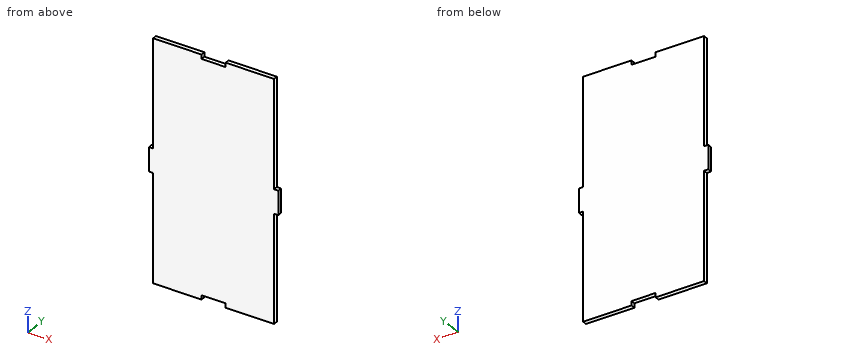
from build123d import *

# Parameters (mm, degrees)
F0_W     = 2.7432
F0_H     = 15.24
F1_DEPTH = 2.7432


with BuildPart() as f1:
    # F0 (on Front) → F1 (new body)
    with BuildSketch(Plane.XZ):
        Polygon((-7.62, 84.245604), (-38.1, 84.245604), (-38.1, 15.665604), (-38.1, 0.425604), (-38.1, -68.154396), (-7.62, -68.154396), (-7.62, -65.411196), (7.62, -65.411196), (7.62, -68.154396), (38.1, -68.154396), (38.1, 0.425604), (38.1, 15.665604), (38.1, 84.245604), (7.62, 84.245604), (7.62, 81.502404), (-7.62, 81.502404), align=None)
        with Locations((-39.4716, 8.045604)):
            Rectangle(F0_W, F0_H)
        with Locations((39.4716, 8.045604)):
            Rectangle(F0_W, F0_H)
    extrude(amount=F1_DEPTH)


solid = f1.part
Model file for the job. Use its own axes, mm. Give positions to 0.01 mm unless a question says otherwise; leave off trailing zeros. Write each loop counter-clockwise with the first axis right and the second up, starting at its lowest first coordinate (ties: lowest second). Pieces come first, ordered by that corner, then holes. Notation, with made-up numbers: M 62.25,0 L 71.25,0 A19 ccw 71.25,26 Z; hole C 38,13.5 d2. An arc over 180 degrees is marked long. One line per item, written item: value. Start each with the question number.
Q1. Drop flat-ended pins along their axis: pin 1 Ø1.5 at (y, z) = (-0.5, 65.5) entering from +X; pin 2 Ø1 at (y, z) = (-1.5, -25) entering from -X; pin 3 Ø1.4 at (x, y) = (39, -2) entering from +Z. Give the stop position or say it passes through.
Q2. Probe probe 1 along X at (y, z) = (-1.75, 40); probe 2 along Z at (x, y) = (2.5, -1.3). List the from-to ranges inside material, lowest first. Write a range as [from, to].
Q3. Saw through at B-B, the plane z = 41.5. Write the cut outline in (x, y).
Q4. Saw through at C-C, the plane x = 1.5. Write the cut outline in (y, z).
Q5. Saw through at A-A, the plane y = -0.7. Write the cut outline in (x, z).
Output values:
1. pin 1: stops at x = 38.1
1. pin 2: stops at x = -38.1
1. pin 3: stops at z = 15.67
2. probe 1: x = [-38.1, 38.1]
2. probe 2: z = [-65.41, 81.5]
3. outline: M -38.1,-2.74 L 38.1,-2.74 L 38.1,0 L -38.1,0 Z
4. outline: M -2.74,-65.41 L 0,-65.41 L 0,81.5 L -2.74,81.5 Z
5. outline: M -40.84,0.43 L -38.1,0.43 L -38.1,-68.15 L -7.62,-68.15 L -7.62,-65.41 L 7.62,-65.41 L 7.62,-68.15 L 38.1,-68.15 L 38.1,0.43 L 40.84,0.43 L 40.84,15.67 L 38.1,15.67 L 38.1,84.25 L 7.62,84.25 L 7.62,81.5 L -7.62,81.5 L -7.62,84.25 L -38.1,84.25 L -38.1,15.67 L -40.84,15.67 Z
